Source: CAD feature listing. Evaluate the final solid. Frame: model axes, mm. A direction names the side the tool comes from. Coordinates: 2 decimals unless noted, no trailing zeros. Order: outer loops, then holes, each group sorted by start corner. A loop starts at its lowest first (then second) coordinate and runs counter-clockwise, first axis right, second up.
```python
from build123d import *

# Parameters (mm, degrees)
SKETCH1_W           = 416.08
SKETCH1_H           = 101.6
BOSS_EXTRUDE2_DEPTH = 254
CUT_EXTRUDE1_DEPTH  = 101.6
SKETCH6_W           = 187.48
SKETCH6_H           = 31.75
CUT_EXTRUDE9_DEPTH  = 251.554
SKETCH8_W           = 327.18
SKETCH8_H           = 12.7
CUT_EXTRUDE11_DEPTH = 228.6
CUT_EXTRUDE12_DEPTH = 498.956952356
CUT_EXTRUDE13_REACH = 493.6
SKETCH10_W          = 162.08
SKETCH10_H          = 13.204649201


with BuildPart() as part:
    # Sketch1 → Boss-Extrude2 (new body)
    with BuildSketch(Plane(origin=(0, 0, 0), x_dir=(1, 0, 0), z_dir=(0, 1, 0))):
        with Locations((208.04, 50.8)):
            Rectangle(SKETCH1_W, SKETCH1_H)
    extrude(amount=BOSS_EXTRUDE2_DEPTH)

    # Sketch2 → Cut-Extrude1 (cut)
    with BuildSketch(Plane.XY):
        Polygon((0, 101.6), (0, 254), (127, 254), align=None)
        Polygon((416.08, 254), (416.08, 101.6), (339.88, 254), align=None)
    extrude(amount=-CUT_EXTRUDE1_DEPTH, mode=Mode.SUBTRACT)

    # Sketch6 → Cut-Extrude9 (cut)
    with BuildSketch(Plane(origin=(0, 0, 0), x_dir=(1, 0, 0), z_dir=(0, 1, 0))):
        with Locations((233.44, 22.225)):
            Rectangle(SKETCH6_W, SKETCH6_H)
    extrude(amount=CUT_EXTRUDE9_DEPTH, mode=Mode.SUBTRACT)

    # Sketch8 → Cut-Extrude11 (cut)
    with BuildSketch(Plane(origin=(0, 254, 0), x_dir=(1, 0, 0), z_dir=(0, 1, 0))):
        with Locations((169.94, 50.8)):
            Rectangle(SKETCH8_W, SKETCH8_H)
        with Locations((169.94, 68.58)):
            Rectangle(SKETCH8_W, SKETCH8_H)
        with Locations((169.94, 86.36)):
            Rectangle(SKETCH8_W, SKETCH8_H)
    extrude(amount=-CUT_EXTRUDE11_DEPTH, mode=Mode.SUBTRACT)

    # Sketch9 → Cut-Extrude12 (cut, through all)
    with BuildSketch(Plane(origin=(416.08, 0, 0), x_dir=(0, 0, -1), z_dir=(1, 0, 0))):
        Polygon((0, 254), (0, 101.6), (38.1, 254), align=None)
    extrude(amount=-CUT_EXTRUDE12_DEPTH, mode=Mode.SUBTRACT)

    # Sketch10 → Cut-Extrude13 (cut, up to next)
    with BuildSketch(Plane.XY.offset(-38.1), mode=Mode.PRIVATE) as cut_extrude13_sk1:
        with Locations((233.44, 17.056383054)):
            Rectangle(SKETCH10_W, SKETCH10_H)
    cut_extrude13_tool1 = extrude(cut_extrude13_sk1.sketch, amount=-CUT_EXTRUDE13_REACH, mode=Mode.PRIVATE) & part.part
    add(cut_extrude13_tool1.solids().sort_by_distance((233.44, 17.056383, -38.1))[0], mode=Mode.SUBTRACT)


solid = part.part
```
Q1. Pull-direction query (Z, two-part tool) for faces 6 (the flat face through (6.35, 68, -51)), 7 (the flat face through (205, 125, -101.6)), 8 (the flat face through (0, 50, -50)); classes: pulls with the +Z half, pulls with the -Z half, needs draft (parallel to the pull), parting line crosses it, or undercut.
Solutions:
face 6: undercut
face 7: pulls with the -Z half
face 8: needs draft
Q2. Section query C-C on x = 186.5. Output: boundary loops of the cut face in (y, z).
Solutions:
outline: (0, -101.6) - (10.45, -101.6) - (10.45, -38.1) - (0, -38.1) - close; (0, -6.35) - (127, -6.35) - (101.6, 0) - (0, 0) - close; (23.66, -101.6) - (254, -101.6) - (254, -92.71) - (25.4, -92.71) - (25.4, -80.01) - (254, -80.01) - (254, -74.93) - (25.4, -74.93) - (25.4, -62.23) - (254, -62.23) - (254, -57.15) - (25.4, -57.15) - (25.4, -44.45) - (254, -44.45) - (254, -38.1) - (251.55, -37.49) - (251.55, -38.1) - (23.66, -38.1) - close
Q3. Material intervals for line 1 along Z through (x, y) = (193.5, 66); line 2 along Z through (x, y) = (166.5, 161.5); line 3 along Z through (x, y) = (17.5, 65), sorted ascending.
Solutions:
line 1: z = -101.6 to -92.71, -80.01 to -74.93, -62.23 to -57.15, -44.45 to -38.1, -6.35 to 0
line 2: z = -101.6 to -92.71, -80.01 to -74.93, -62.23 to -57.15, -44.45 to -38.1
line 3: z = -101.6 to -92.71, -80.01 to -74.93, -62.23 to -57.15, -44.45 to 0
Q4. Section query D-D on y = 203. Output: boundary loops of the cut face in (x, z), plus the area to 3 significant figures.
Solutions:
outline: (84.5, -101.6) - (365.38, -101.6) - (365.38, -25.35) - (327.18, -25.35) - (327.18, -38.1) - (139.7, -38.1) - (139.7, -25.35) - (84.5, -25.35) - (84.5, -44.45) - (333.53, -44.45) - (333.53, -57.15) - (84.5, -57.15) - (84.5, -62.23) - (333.53, -62.23) - (333.53, -74.93) - (84.5, -74.93) - (84.5, -80.01) - (333.53, -80.01) - (333.53, -92.71) - (84.5, -92.71) - close
area: 9,540 mm2
Q5. Section query A-A on z = -31.5. Output: boundary loops of the cut face in (x, y), plus the area to 3 significant figures.
Solutions:
outline: (0, 0) - (139.7, 0) - (139.7, 227.6) - (105, 227.6) - (0, 101.6) - close; (327.18, 0) - (416.08, 0) - (416.08, 101.6) - (353.08, 227.6) - (327.18, 227.6) - close
area: 41,400 mm2
Q6. Set-up query: faces 1 (the flat face through (232, 23.659, -69)), 2 (the flat face through (168, 141, -74.93)), 3 (the flat face through (232, 124, -38.1)), 4 (the flat face through (205, 0, -63)), 5 (the flat face through (232, 63, -6.35)). Return all of +Z, -Z, +X, -X, +Y, -Y with unobstructed straight access to the full face (end or side cutting, diameter ignored); none if empty.
Solutions:
face 1: -Z
face 2: +Y
face 3: -Y
face 4: +Z, -Z, +X, -X, -Y
face 5: +Y, -Y
Q7. Section query B-B on y = 56.5. Output: boundary loops of the cut face in (x, z), plus the area to 3 significant figures.
Solutions:
outline: (0, -101.6) - (416.08, -101.6) - (416.08, 0) - (0, 0) - close; hole (6.35, -92.71) - (333.53, -92.71) - (333.53, -80.01) - (6.35, -80.01) - close; hole (6.35, -74.93) - (333.53, -74.93) - (333.53, -62.23) - (6.35, -62.23) - close; hole (6.35, -57.15) - (333.53, -57.15) - (333.53, -44.45) - (6.35, -44.45) - close; hole (139.7, -38.1) - (327.18, -38.1) - (327.18, -6.35) - (139.7, -6.35) - close
area: 23,900 mm2
Q8. Pin query (flat end, axial travel): P1, Ø8, axis at y = 192.5, z = -56.5, coming from the +X side; P2, Ø2, axis at y = 108.5, z = -33.5, coming from the -X side; P3, Ø10, axis at x = 214.5, z = -67.5, coming from the +Y side. Return the tip coordinate at first contact, or that it passes through.
Solutions:
P1: stops at x = 372.63
P2: stops at x = 4.92
P3: stops at y = 25.4
